The model under review builds one solid part; all positions refer to its coordinate system, in mm. Face numbers are marked on the shaded views. A direction names the side the tool comes from. Round coordinates to 2 decimals unless told otherwise and drop trailing zeros. Write each loop counter-clockwise with the first axis right and the second up, starting at its lowest first coordinate (ties: lowest second). Pieces come first, ordered by that corner, then holes. Notation, with made-up numbers: (83.5, 3) - (135.5, 3) arc R24 ccw to (135.5, 40) - close; hole circle Ø1 at (15, 76). An arc over 180 degrees is marked (long way). Write each question's results on one line, items separated by ' | '.
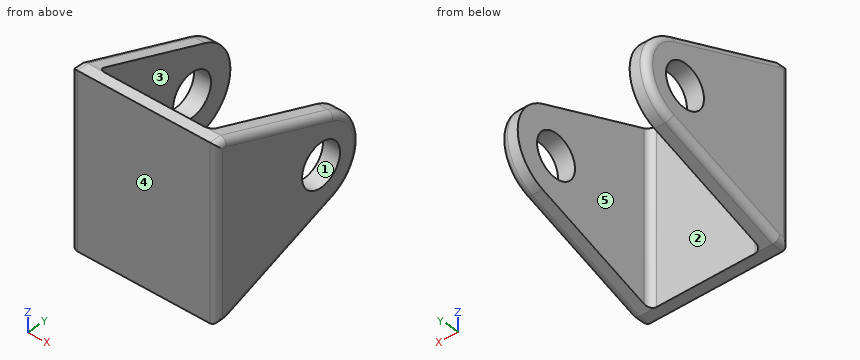
Autodesk Inventor part; units mm, degrees
ref_plane "YZ Plane" through (0, 0, 0) normal (1, 0, 0) x (0, 1, 0)
ref_plane "XZ Plane" through (0, 0, 0) normal (0, 1, 0) x (-1, 0, 0)
ref_plane "XY Plane" through (0, 0, 0) normal (0, 0, 1) x (1, 0, 0)
sketch "Sketch1" plane through (0, 0, 0) normal (1, 0, 0) x (0, 1, 0)
  circle A0 centre (0, 0) radius 6.35
  line L0 (0, 0) -> (-34.925, 0)
  line L1 (-34.925, 25.4) -> (-34.925, -25.4)
  line L2 (-34.925, 25.4) -> (-31.425, 25.4)
  line L3 (-31.425, 25.4) -> (-31.425, -25.4)
  line L4 (-31.425, -25.4) -> (-34.925, -25.4)
  line L5 (-34.925, -25.4) -> (-34.925, 25.4)
  circle A1 centre (0, 0) radius 12.827
  line L6 (4.4793, 12.0195) -> (-31.425, 25.4)
  line L7 (4.4793, -12.0195) -> (-31.425, -25.4)
  dimension "d0" = 12.7
  dimension "d1" = 34.925
  dimension "d2" = 50.8
  dimension "d3" = 3.5
  dimension "d4" = 25.654
extrude "Extrusion1" add sketch "Sketch1" along normal blind 43.4975 contours L3 L4 L1 L0 | L0 L1 L2 L3
sketch "Sketch2" plane through (43.4975, 0, 0) normal (1, 0, 0) x (0, 0, -1)
  line L0 (-25.4, -34.925) -> (25.4, -34.925)
  line L1 (25.4, -34.925) -> (25.4, -31.425)
  line L2 (25.4, -31.425) -> (-25.4, -31.425)
  line L3 (-25.4, -31.425) -> (-25.4, -34.925)
  line L4 (-25.4, -31.425) -> (-25.4, -34.925)
  line L5 (-25.4, -34.925) -> (25.4, -34.925)
  line L6 (-25.4, -31.425) -> (-25.4, -34.925)
  line L7 (25.4, -31.425) -> (-25.4, -31.425)
  line L8 (25.4, -34.925) -> (25.4, -31.425)
  line L9 (-25.4, -31.425) -> (-25.4, -34.925)
  line L10 (-25.4, -31.425) -> (-25.4, -34.925)
  circle A0 centre (0, 0) radius 6.35
  line L11 (0, 0) -> (0, -34.925)
  line L12 (-25.4, -34.925) -> (25.4, -34.925)
  line L13 (-25.4, -34.925) -> (-25.4, -31.425)
  line L14 (-25.4, -31.425) -> (25.4, -31.425)
  line L15 (25.4, -31.425) -> (25.4, -34.925)
  line L16 (25.4, -34.925) -> (-25.4, -34.925)
  circle A1 centre (0, 0) radius 12.827
  line L17 (-12.0195, 4.4793) -> (-25.4, -31.425)
  line L18 (12.0195, 4.4793) -> (25.4, -31.425)
extrude "Extrusion2" add sketch "Sketch1" along normal blind 5.08 contours A1 | A1 L7 L3 L0 | L0 L3 L6 A1
extrude "Extrusion3" add sketch "Sketch2" against normal blind 5.08 contours L17 A1 L11 L2 | L11 A1 L18 L2 | A1
fillet "Fillet1" radius 2 14 edges at (43.4975, 12.827, 0) (43.4975, -13.4728, -18.7097) (43.4975, -13.4728, 18.7097) (0, 12.827, 0) (0, -13.4728, -18.7097) (0, -13.4728, 18.7097) (43.4975, -33.175, 25.4) (43.4975, -33.175, -25.4) (0, -33.175, 25.4) (0, -33.175, -25.4) (43.4975, -34.925, 0) (0, -34.925, 0) (38.4175, -31.425, 0) (5.08, -31.425, 0)
properties part number "largebracket"
Q1. We need section D-D (x = 31). State the section outline as (y, z) points (3 decimals).
Evaluation:
outline: (-34.925, -25.4) - (-31.425, -25.4) - (-31.425, 25.4) - (-34.925, 25.4) - close
Q2. For probe 1 along X at (y, z) = (-7, -12); probe 2 along Y at (x, z) = (20.5, -5) (3 decimals); probe 3 along Z at (x, y) = (3.3, 0), list the stretches that pass through material, from the lowest coordinate up.
Evaluation:
probe 1: x = 0 to 5.08, 38.42 to 43.5 | probe 2: y = -34.925 to -31.425 | probe 3: z = -13.69 to -6.35, 6.35 to 13.69
Q3. The part is to be moulded in two halves that separate along Y. For the marked faces 1, 2 and 3, say which applies: released by +Y, released by -Y, zero draft, split by the parting line, or undercut.
Evaluation:
face 1: undercut | face 2: released by +Y | face 3: zero draft
Q4. Insertion check: P1, Ø11.5, axis at y = 0, z = 0, coming from the +X side; P2, Ø5, axis at x = 30, z = 6, coming from the +Y side (3 decimals); P3, Ø6, axis at x = 5.5, y = -10.5, coming from the -Z side. Each pin has a flat end and moves straight along its axis. Give the tip position at first contact, or say it passes through.
Evaluation:
P1: passes through | P2: stops at y = -31.425 | P3: stops at z = -18.71
Q5. Tool access review of the marked faces 4 and 5: name each direction out of +Z, -Z, +X, -X, +Y, -Y from which nothing blocks a thin tool from reaching the whole face with its end or side.
Evaluation:
face 4: +Z, -Z, +X, -X, -Y | face 5: +Z, -Z, +Y
Q6. We need section A-A (z = 0). State how many separate pieces and enclosed holes the cut face has, plus the area to 3 significant figures.
Evaluation:
separate pieces: 3 | enclosed holes: 0 | area: 471 mm^2
